The listing builds one solid part. Answer for the finished solid, in the listing's coordinates (mm). Face numbers are marked on the shaded views. Round coordinates to 2 decimals unless told otherwise and drop trailing zeros. Order: outer loops, then holes, each group sorted by start corner. A loop starts at its lowest first (then second) coordinate and runs counter-clockwise, first axis right, second up. Notation, with made-up numbers: M 52,-3.75 L 65,-3.75 A28 cw 65,21.25 Z; hole C 33,7 d1. An arc over 180 degrees is marked long. Put each result on its own line as item: value. Start each with the question number.
1. The part is cut by section A-A (z = 5.5). Give the vertices of the cut face in (x, y), then the cut area to 3 significant figures.
2. Consider line 1 (Y direction, x = 152, z = 1.4); line 2 (Y direction, x = 29, z = 0.7); line 3 (X direction, y = 60, z = 3.75). Determine where each line is inside the solid, lowest interval first.
3. The part is cut by section B-B (x = 152). Give the vertices of the cut face in (y, z).
4. The part is cut by section C-C (y = 88.5). Give the vertices of the cut face in (x, z), then the cut area to 3 significant figures.
5. The mould has two halves that part along X. Classify the marked faces 1, 2 and 3: +X half, -X half, draft (parallel to the pull), parting line (faces both ways), or undercut.
6. The part is cut by section D-D (x = 29). Give the vertices of the cut face in (y, z), then the cut area to 3 significant figures.
7. Each of these flat-tipped pins is pushed along its axis until it touches: pin 1 Ø6.5 at (x, z) = (188.5, 8) entering from +Y; pin 2 Ø5.5 at (x, y) = (15, 61.5) entering from +Z; pin 3 Ø4 at (x, z) = (187, 7.5) entering from -Y; pin 4 Ø3 at (y, z) = (59.5, 6.5) entering from +X. Where does it stop, or does it pass through?
from build123d import *

# Parameters (mm, degrees)
BOX_W             = 211
BOX_H             = 198
BOX_DEPTH         = 2
BOX001_W          = 186
BOX001_H          = 89
BOX001_DEPTH      = 10
BOX002_W          = 184
BOX002_H          = 87
BOX002_DEPTH      = 10
BOX003_W          = 160
BOX003_H          = 89
BOX003_DEPTH      = 10
CYLINDER_R        = 16
CYLINDER_DEPTH    = 2
CYLINDER001_R     = 25
CYLINDER001_DEPTH = 2
CYLINDER002_R     = 17
CYLINDER002_DEPTH = 20
CYLINDER003_R     = 16
CYLINDER003_DEPTH = 20
CYLINDER004_R     = 37
CYLINDER004_DEPTH = 2


with BuildPart() as part:
    # Box → Box (join)
    with BuildSketch(Plane.XY):
        with Locations((105.5, 99)):
            Rectangle(BOX_W, BOX_H)
    extrude(amount=BOX_DEPTH)

    # Box001 → Box001 (join)
    with BuildSketch(Plane(origin=(9, 10, 0), x_dir=(1, 0, 0), z_dir=(0, 0, 1))):
        with Locations((93, 44.5)):
            Rectangle(BOX001_W, BOX001_H)
    extrude(amount=BOX001_DEPTH)

    # Box002 → Box002 (cut)
    with BuildSketch(Plane(origin=(10, 11, 0), x_dir=(1, 0, 0), z_dir=(0, 0, 1))):
        with Locations((92, 43.5)):
            Rectangle(BOX002_W, BOX002_H)
    extrude(amount=BOX002_DEPTH, mode=Mode.SUBTRACT)

    # Box003 → Box003 (cut)
    with BuildSketch(Plane(origin=(20, 10, 2), x_dir=(1, 0, 0), z_dir=(0, 0, 1))):
        with Locations((80, 44.5)):
            Rectangle(BOX003_W, BOX003_H)
    extrude(amount=BOX003_DEPTH, mode=Mode.SUBTRACT)

    # Cylinder → Cylinder (cut)
    with BuildSketch(Plane(origin=(29, 127, 0), x_dir=(1, 0, 0), z_dir=(0, 0, 1))):
        Circle(CYLINDER_R)
    extrude(amount=CYLINDER_DEPTH, mode=Mode.SUBTRACT)

    # Cylinder001 → Cylinder001 (cut)
    with BuildSketch(Plane(origin=(82, 135, 0), x_dir=(1, 0, 0), z_dir=(0, 0, 1))):
        Circle(CYLINDER001_R)
    extrude(amount=CYLINDER001_DEPTH, mode=Mode.SUBTRACT)

    # Cylinder002 → Cylinder002 (join)
    with BuildSketch(Plane(origin=(29, 166, 0), x_dir=(1, 0, 0), z_dir=(0, 0, 1))):
        Circle(CYLINDER002_R)
    extrude(amount=CYLINDER002_DEPTH)

    # Cylinder003 → Cylinder003 (cut)
    with BuildSketch(Plane(origin=(29, 166, 0), x_dir=(1, 0, 0), z_dir=(0, 0, 1))):
        Circle(CYLINDER003_R)
    extrude(amount=CYLINDER003_DEPTH, mode=Mode.SUBTRACT)

    # Cylinder004 → Cylinder004 (cut)
    with BuildSketch(Plane(origin=(152, 150, 0), x_dir=(1, 0, 0), z_dir=(0, 0, 1))):
        Circle(CYLINDER004_R)
    extrude(amount=CYLINDER004_DEPTH, mode=Mode.SUBTRACT)


solid = part.part
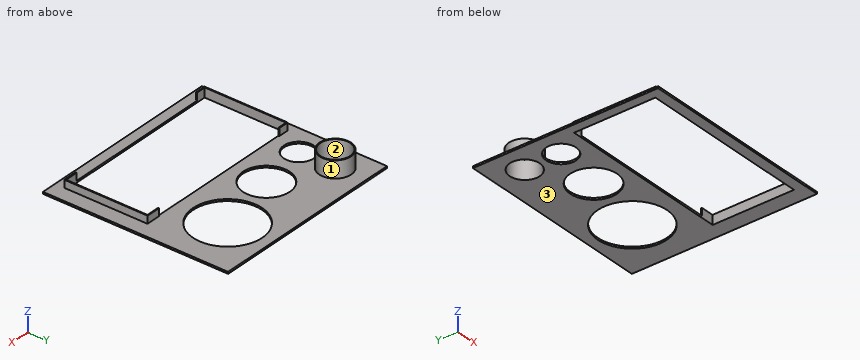
Resolved:
1. outline: M 9,10 L 20,10 L 20,11 L 10,11 L 10,98 L 20,98 L 20,99 L 9,99 Z; C 29,166 d34; M 180,10 L 195,10 L 195,99 L 180,99 L 180,98 L 194,98 L 194,11 L 180,11 Z; hole C 29,166 d32
1. area: 330 mm2
2. line 1: 0 to 11, 98 to 113, 187 to 198
2. line 2: 0 to 11, 98 to 111, 143 to 150, 182 to 198
2. line 3: 9 to 10, 194 to 195
3. outline: M 0,0 L 11,0 L 11,2 L 0,2 Z; M 98,0 L 113,0 L 113,2 L 98,2 Z; M 187,0 L 198,0 L 198,2 L 187,2 Z
4. outline: M 0,0 L 10,0 L 10,10 L 9,10 L 9,2 L 0,2 Z; M 194,0 L 211,0 L 211,2 L 195,2 L 195,10 L 194,10 Z
4. area: 70.0 mm2
5. face 1: parting line
5. face 2: undercut
5. face 3: draft
6. outline: M 0,0 L 11,0 L 11,2 L 0,2 Z; M 98,0 L 111,0 L 111,2 L 98,2 Z; M 143,0 L 150,0 L 150,20 L 149,20 L 149,2 L 143,2 Z; M 182,0 L 198,0 L 198,2 L 183,2 L 183,20 L 182,20 Z
6. area: 130 mm2
7. pin 1: y = 99
7. pin 2: through
7. pin 3: y = 10
7. pin 4: x = 195
